For this review, take the finished solid that the model builds, in its own axes (mm). Face numbers are marked on the shaded views. Coordinates: 2 decimals unless noted, no trailing zeros. Write each loop counter-clockwise with the first axis right and the second up, starting at its lowest first coordinate (ties: lowest second). Pieces come first, ordered by that corner, then holes. Notation, with made-up numbers: M -14.75,-35.5 L 5.25,-35.5 A26 ccw 5.25,-12.5 Z; hole C 79,11.25 d1. An arc over 180 degrees is marked long. One line per question, with ' | ' between items.
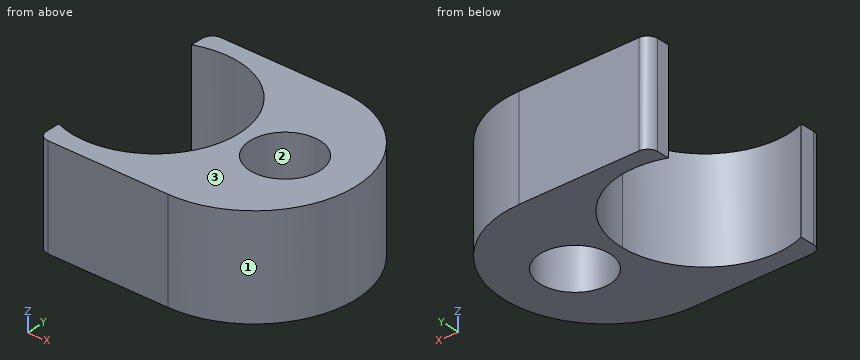
from build123d import *

# Parameters (mm, degrees)
F0_R     = 6.9
F1_DEPTH = 20
F3_R     = 2


# Not quite as in the source:
# - a feature of the source that left no trace in its solid (it failed there, or was rolled back) is left out


with BuildPart() as f1:
    # F0 (on Top) → F1 (new body)
    with BuildSketch(Plane.XY):
        with BuildLine():
            ThreePointArc((-6, 15.3704261489), (9.3072552345, 13.6244265934), (16.5, 0))
            ThreePointArc((16.5, 0), (9.3072552345, -13.6244265934), (-6, -15.3704261489))
            Line((-6, -15.3704261489), (-6, -20.1503510079))
            Line((-6, -20.1503510079), (-6, -20.1573419994))
            Line((-6, -20.1573419994), (19.9984760751, -20.1573419994))
            ThreePointArc((19.9984760751, -20.1573419994), (40.0019715709, -0.1538465036), (19.9984760751, 19.8496489921))
            Line((19.9984760751, 19.8496489921), (-6, 19.8496489921))
            Line((-6, 19.8496489921), (-6, 15.3704261489))
        make_face()
        with Locations((26, 0)):
            Circle(F0_R, mode=Mode.SUBTRACT)
    extrude(amount=F1_DEPTH)

    # F3
    f3_edges = [f1.edges().sort_by_distance(p)[0] for p in [
        (-6, -20.157342, 10),
        (-6, 19.849649, 10),
    ]]
    fillet(f3_edges, radius=F3_R)


solid = f1.part
1) We need section A-A on z = 2.25. State the section outline as (x, y) points, then the cut area to 3 significant figures.
Responses:
outline: M -6,-18.16 A2 ccw -4,-20.16 L 20,-20.16 A20 ccw 20,19.85 L -4,19.85 A2 ccw -6,17.85 L -6,15.37 A16.5 cw long -6,-15.37 Z; hole C 26,0 d13.8 | area: 896 mm^2
2) To check wall thickness, follow line 1 along Y through (x, z) = (26, 10.25); line 2 along X through (y, z) = (5.5, 6.5); line 3 along Y through (x, z) = (-1, 4.5). State the ranges of each line that lie inside material, in increasing order. Write a range as [from, to].
Responses:
line 1: [-19.24, -6.9], [6.9, 18.93] | line 2: [15.56, 21.83], [30.17, 39.19] | line 3: [-20.16, -16.47], [16.47, 19.85]
3) We need section D-D on x = 36. State the section outline as (y, z) points, then the cut area to 3 significant figures.
Responses:
outline: M -12.16,0 L 11.85,0 L 11.85,20 L -12.16,20 Z | area: 480 mm^2
4) We need section B-B on x = 2. State the section outline as (y, z) points, then the cut area to 3 significant figures.
Responses:
outline: M -20.16,0 L -16.38,0 L -16.38,20 L -20.16,20 Z; M 16.38,0 L 19.85,0 L 19.85,20 L 16.38,20 Z | area: 145 mm^2
5) Insertion check: pin 1 Ø12 at (x, z) = (31, 2.5) entering from -Y; pin 2 Ø16 at (x, y) = (26, 0) entering from +Z; pin 3 Ø1.5 at (y, z) = (-6.5, 5) entering from -X; pin 4 Ø6 at (y, z) = (2, 5.5) entering from -X. Each pin has a flat end and moves straight along its axis. Give the tip position at first contact, or say it passes through.
Responses:
pin 1: y = -19.52 | pin 2: z = 20 | pin 3: x = 14.82 | pin 4: x = 15.72
6) The part is to be moulded in two halves that separate along X. For the marked faces 1, 2 and 3, say which applies: +X half, -X half, draft (parallel to the pull), parting line (faces both ways), or undercut.
Responses:
face 1: +X half | face 2: undercut | face 3: draft
7) We need section C-C on y = -6. State the section outline as (x, z) points, then the cut area to 3 significant figures.
Responses:
outline: M 15.37,0 L 22.59,0 L 22.59,20 L 15.37,20 Z; M 29.41,0 L 39.13,0 L 39.13,20 L 29.41,20 Z | area: 339 mm^2
